from build123d import *

# Parameters (mm, degrees)
F0_R     = 61.50483
F0_R_2   = 48.80483
F1_DEPTH = 38.1
F2_DEPTH = 12.7
F3_D     = 13.49248
F3_DEPTH = 31.2674
F3_TIP   = 4.0535499425
F4_SIZE  = 1.524


with BuildPart() as f1:
    # F0 (on Front) → F1 (new body)
    with BuildSketch(Plane.XZ):
        Circle(F0_R)
        Circle(F0_R_2, mode=Mode.SUBTRACT)
    extrude(amount=F1_DEPTH)

    # F0 (on Front) → F2 (join)
    with BuildSketch(Plane.XZ):
        Circle(F0_R)
        Circle(F0_R_2, mode=Mode.SUBTRACT)
        Circle(F0_R_2)
    extrude(amount=-F2_DEPTH)

    # F3
    with Locations(Plane.XZ):
        with Locations((0, 0)):
            Hole(F3_D / 2, depth=F3_DEPTH)
            with Locations((0, 0, -(F3_DEPTH + F3_TIP / 2))):  # 118° drill point
                Cone(0, F3_D / 2, F3_TIP, mode=Mode.SUBTRACT)

    # F4
    f4_edges = [f1.edges().sort_by_distance(p)[0] for p in [
        (61.50483, -19.05, 0),
        (-61.50483, 0, 0),
        (-61.50483, -38.1, 0),
        (61.50483, 6.35, 0),
        (-61.50483, 12.7, 0),
        (48.80483, -19.05, 0),
        (-48.80483, 0, 0),
        (-48.80483, -38.1, 0),
    ]]
    chamfer(f4_edges, length=F4_SIZE)


solid = f1.part
The listing builds one solid part. Answer for the finished solid, in the listing's coordinates (mm). A direction names the side the tool comes from. Give positions to 0.01 mm unless a question says otherwise; leave off trailing zeros. Order: outer loops, then holes, each group sorted by start corner. A loop starts at its lowest first (then second) coordinate and runs counter-clockwise, first axis right, second up. Notation, with made-up numbers: (4, 23.5) - (59, 23.5) arc R5 cw to (59, 29.5) - close; hole circle Ø7 at (-37, -35). An arc over 180 degrees is marked (long way). One line per item, written item: value. Start each with the question number.
1) A cutting plane is placed at A-A on z = 0. Give the vertices of the cut face in (x, y), then the cut area to 3 significant figures.
2) The mould has two halves that part along Z. Classify faces 3 (the face through (-1, 0, -10)), 4 (the face through (-48.81, -13.03, -37.42)), 5 (the face through (-6.435, 6.439, 2.026)), 6 (the face through (-14, -38.1, 49)): released by +Z, released by -Z, zero draft, split by the parting line, or undercut.
3) A cutting plane is placed at C-C on y = -13. Give the vertices of the cut face in (x, z).
4) Given pin 1 Ø10 at (x, y) = (44.5, -4) entering from +Z; pin 2 Ø8 at (y, z) = (7.5, -5.5) entering from +X; pin 3 Ø1.5 at (x, y) = (-38, -19.5) entering from -Z, each flat-ended and moving along its own axis, determine where each tip first touches the part or whether it passes through.
5) A cutting plane is placed at B-B on x = 0. Give the vertices of the cut face in (y, z), then the cut area to 3 significant figures.
6) A tool of negligible diameter and unlimited length cuts with its end or side. For faces 1 (the face through (-10.58, -18.805, -47.644)), 2 (the face through (12, 12.7, 1)), from which of +Z, -Z, +X, -X, +Y, -Y can it reach the whole face along a straight path? Write none if from no direction.
7) Find the intervals of material crossed by L1, parallel to Z at x = 0, y = -14.5; L2, parallel to Y at x = -30.5, z = -10, in increasing order.
Answer sheet:
1. outline: (-61.5, -36.58) - (-59.98, -38.1) - (-50.33, -38.1) - (-48.8, -36.58) - (-48.8, -1.52) - (-47.28, 0) - (-6.75, 0) - (-6.75, 12.7) - (-59.98, 12.7) - (-61.5, 11.18) - close; (6.75, 0) - (47.28, 0) - (48.8, -1.52) - (48.8, -36.58) - (50.33, -38.1) - (59.98, -38.1) - (61.5, -36.58) - (61.5, 11.18) - (59.98, 12.7) - (6.75, 12.7) - close
1. area: 2,350 mm2
2. face 3: undercut
2. face 4: split by the parting line
2. face 5: undercut
2. face 6: zero draft
3. outline: circle Ø123.01 at (0, 0); hole circle Ø97.61 at (0, 0)
4. pin 1: stops at z = 47.14
4. pin 2: stops at x = 61.49
4. pin 3: stops at z = -48.94
5. outline: (-38.1, -59.98) - (-36.58, -61.5) - (11.18, -61.5) - (12.7, -59.98) - (12.7, -6.75) - (0, -6.75) - (0, -47.28) - (-1.52, -48.8) - (-36.58, -48.8) - (-38.1, -50.33) - close; (-38.1, 50.33) - (-36.58, 48.8) - (-1.52, 48.8) - (0, 47.28) - (0, 6.75) - (12.7, 6.75) - (12.7, 59.98) - (11.18, 61.5) - (-36.58, 61.5) - (-38.1, 59.98) - close
5. area: 2,350 mm2
6. face 1: -Y
6. face 2: +Z, -Z, +X, -X, +Y
7. L1: z = -61.5 to -48.8, 48.8 to 61.5
7. L2: y = 0 to 12.7
